Can you work these out from the drawing? Everything is in mm from the part's minimum corner. A direction names the side the tool comes from. Coordinates: 2 decimals unless noted, no trailing zeros. Order: outer loops, then holes, each group sorted by start corner. A loop starts at its lowest first (then second) coordinate and runs counter-clockwise, first axis right, second up. Notation, with made-up numbers: (11, 6.25) -> (39, 6.25) arc R14 ccw to (39, 11.25) -> close; hole circle Ø9 at (-36, 5). An arc over 180 degrees is marked (long way). Write item = value, one per line. Start each with the question number.
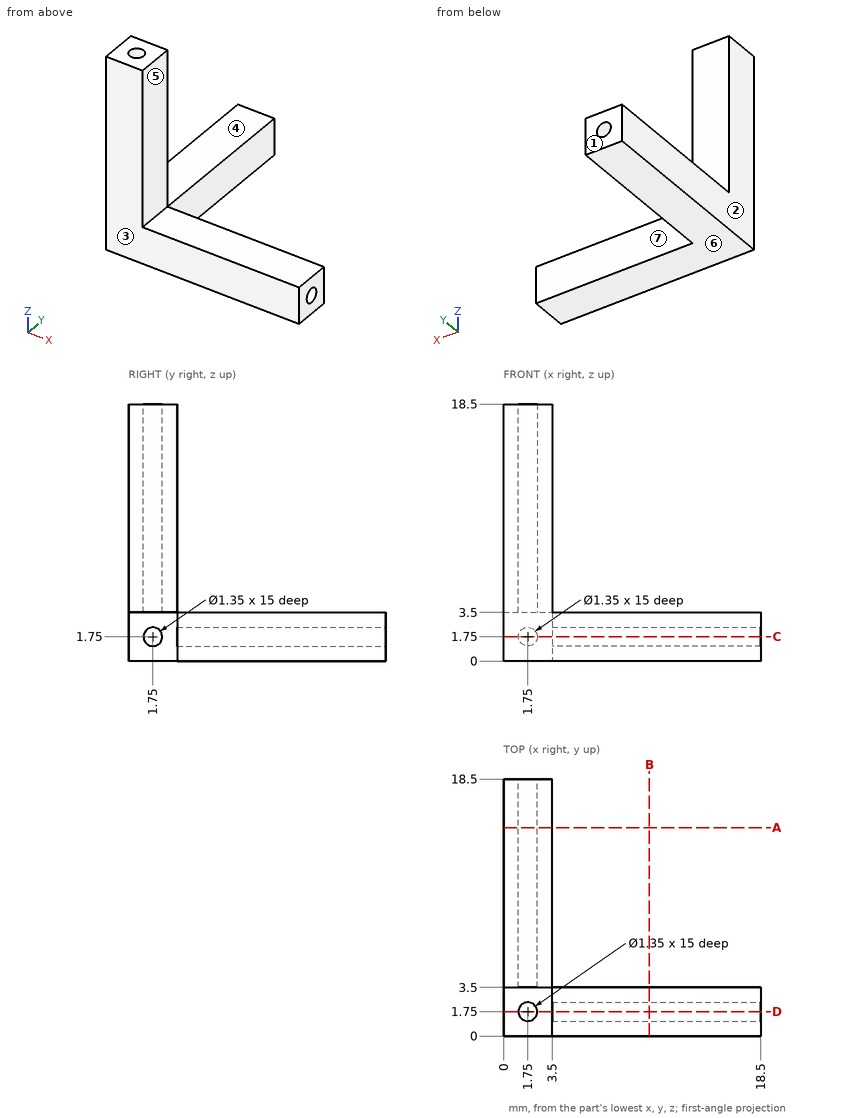
(1) For P1, Ø1.8, axis at y = 9.5, z = 1, coming from the +X side; P2, Ø1, axis at x = 11.5, z = 2.5, coming from the +Y side; P3, Ø1, axis at x = 10, y = 2.5, coming from the +Z side; P4, Ø5, axis at x = 16.5, y = 2.5, coming from the -Z side, each with a flat end and sliding along its axis, tell me the tip position at first contact or that it passes through.
(2) If I drill on L1, parallel to Z at x = 1.75, y = 7.25 (3 decimals); L2, parallel to Y at x = 3.25, z = 17.75, over which ranges is the centre line in solid material (lowest first)? Write a range as from..to.
(3) Imagine slicing it at A-A (y = 15). Write out the boundary of the cut face in (x, z) (3 decimals), plus the area to 3 significant figures.
(4) For the marked faces 4, 5, 6 and 7, which set-ups out of +Z, -Z, +X, -X, +Y, -Y let a thin tool reach every point of the face, with its end or its side?
(5) Imagine slicing it at C-C (z = 1.75). Write out the boundary of the cut face in (x, y) (3 decimals).
(6) Thinking about a two-plate mould opening in Y: for the marked faces 1, 2 and 3, which applies, +Y half, -Y half, draft (parallel to the pull), parting line (faces both ways), or undercut?
Result set:
q1.P1 = 3.5
q1.P2 = 3.5
q1.P3 = 3.5
q1.P4 = 0
q2.L1 = 0..1.075, 2.425..3.5
q2.L2 = 0..3.5
q3.outline = (0, 0) -> (3.5, 0) -> (3.5, 3.5) -> (0, 3.5) -> close; hole circle Ø1.35 at (1.75, 1.75)
q3.area = 10.8 mm2
q4.face_4 = +Z, +X, -X, +Y
q4.face_5 = +Z, +X, +Y, -Y
q4.face_6 = -Z, +X, -X, +Y, -Y
q4.face_7 = +Z, -Z, +X, +Y
q5.outline = (0, 0) -> (18.5, 0) -> (18.5, 1.075) -> (3.5, 1.075) -> (3.5, 2.425) -> (18.5, 2.425) -> (18.5, 3.5) -> (3.5, 3.5) -> (3.5, 18.5) -> (2.425, 18.5) -> (2.425, 3.5) -> (1.075, 3.5) -> (1.075, 18.5) -> (0, 18.5) -> close
q6.face_1 = +Y half
q6.face_2 = draft
q6.face_3 = -Y half
